Part print with two shaded views. Sizes in mm from the minimum x, y, z corner. A direction names the side the tool comes from. Round coordinates to 2 decimals unless told otherwise and drop trailing zeros. Order: outer loops, then holes, each group sorted by start corner. A loop starts at its lowest first (then second) coordinate and runs counter-clockwise, first axis right, second up. Notation, with made-up numbers: M 57.25,34 L 73.25,34 A19 cw 73.25,64 Z; hole C -30,15 d11. An arc over 180 degrees is marked long. Answer as a JSON object with one key per item and string values.
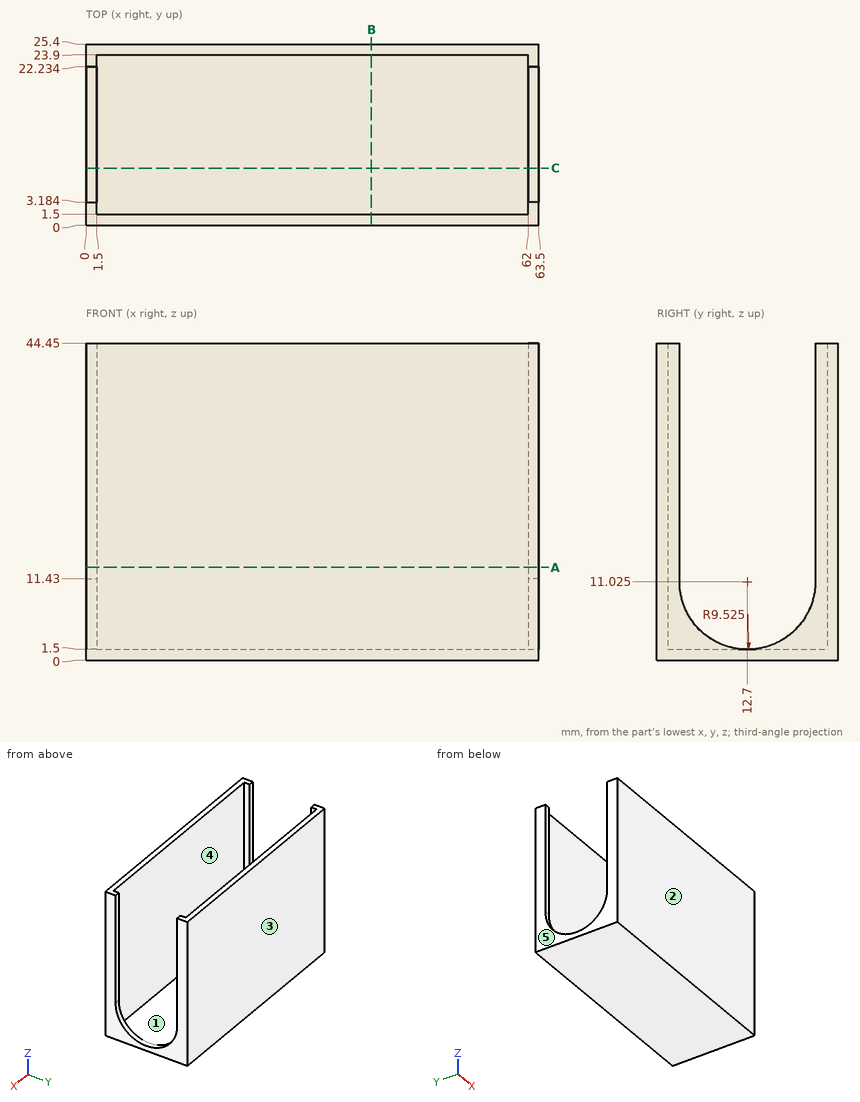
Item 1: 3-axis set-ups, long thin cutter, end or side, ignore diameter. For the marked faces 1 and 2: which of +Z, -Z, +X, -X, +Y, -Y reach the whole face in a straight line?
Worked answers:
{"face 1": "+Z", "face 2": "+Z, -Z, +X, -X, -Y"}
Item 2: Saw through at A-A on z = 13. List the corners of the cut face in (x, y).
Worked answers:
{"outline": "M 0,0 L 63.5,0 L 63.5,3.18 L 62,3.18 L 62,1.5 L 1.5,1.5 L 1.5,3.18 L 0,3.18 Z; M 0,22.23 L 1.5,22.23 L 1.5,23.9 L 62,23.9 L 62,22.23 L 63.5,22.23 L 63.5,25.4 L 0,25.4 Z"}
Item 3: Wall check: line 1 along Y through (x, z) = (4, 41.5); line 2 along Z through (x, y) = (23, 19.75). Give the ranges that are in metal, low to high. Write a range as [from, to].
Worked answers:
{"line 1": "y = [0, 1.5], [23.9, 25.4]", "line 2": "z = [0, 1.5]"}
Item 4: Saw through at C-C on y = 8. List the corners of the cut face in (x, z).
Worked answers:
{"outline": "M 0,0 L 63.5,0 L 63.5,2.74 L 62,2.74 L 62,1.5 L 1.5,1.5 L 1.5,2.74 L 0,2.74 Z"}
Item 5: Two-plate mould, pull along Y, no slides. Class the marked faces 3, 4 and 5: released by +Y, released by -Y, zero draft, split by the parting line, or undercut.
Worked answers:
{"face 3": "released by +Y", "face 4": "undercut", "face 5": "zero draft"}
Item 6: Saw through at B-B on x = 40. List the corners of the cut face in (y, z), and give its area (3 significant figures).
Worked answers:
{"outline": "M 0,0 L 25.4,0 L 25.4,44.45 L 23.9,44.45 L 23.9,1.5 L 1.5,1.5 L 1.5,44.45 L 0,44.45 Z", "area": "167 mm2"}
Item 7: Drop flat-ended pins along their axis: pin 1 Ø5 at (x, y) = (10.5, 4) entering from -Z; pin 2 Ø1 at (x, y) = (44, 9) entering from +Z; pin 3 Ø5.5 at (y, z) = (17.5, 29) entering from -X. Give the stop position or say it passes through.
Worked answers:
{"pin 1": "stops at z = 0", "pin 2": "stops at z = 1.5", "pin 3": "passes through"}
